```python
from build123d import *

# Parameters (mm, degrees)
SKETCH1_R           = 7.5
SKETCH1_R_2         = 3
BOSS_EXTRUDE1_DEPTH = 12.7


with BuildPart() as part:
    # Sketch1 → Boss-Extrude1 (new body)
    with BuildSketch(Plane(origin=(0, 0, 0), x_dir=(1, 0, 0), z_dir=(0, 1, 0))):
        with BuildLine():
            Line((4.628728323, 75), (-4.628728323, 75))
            ThreePointArc((-4.628728323, 75), (-8.298056729, 73.747212766), (-10.435089207, 70.512009682))
            add(Edge.make_bspline(
                [(-10.435089207, 70.512009682), (-11.436889623, 66.664934619), (-14.691827535, 59.170334198), (-20.319154818, 53.251718644), (-23.989109736, 50.544662785)],
                knots=[0.130554933, 0.130554933, 0.130554933, 0.130554933, 0.477565762, 0.872598063, 0.872598063, 0.872598063, 0.872598063], degree=3))
            ThreePointArc((-23.989109736, 50.544662785), (-26.161679176, 47.482134252), (-26.088483789, 43.727965713))
            add(Edge.make_bspline(
                [(-26.088483789, 43.727965713), (-23.983802584, 37.735198712), (-21.861167747, 26.954437426), (-23.911988058, 18.58322157), (-25.980762, 15)],
                knots=[0.052697527, 0.052697527, 0.052697527, 0.052697527, 0.276348764, 0.5, 0.5, 0.5, 0.5], degree=3))
            add(Edge.make_bspline(
                [(-50.913771074, 0.729306865), (-44.671541988, 1.902983), (-34.273811388, 5.455107991), (-28.049535938, 11.416778424), (-25.980762, 15)],
                knots=[0.052697527, 0.052697527, 0.052697527, 0.052697527, 0.276348763, 0.5, 0.5, 0.5, 0.5], degree=3))
            ThreePointArc((-50.913771074, 0.729306865), (-54.201574082, -1.084388344), (-55.767516863, -4.497152931))
            add(Edge.make_bspline(
                [(-66.282736261, -26.218952497), (-63.451971733, -23.427830356), (-58.58892633, -16.861671221), (-56.276918547, -9.028955057), (-55.767516863, -4.497152931)],
                knots=[0.130554933, 0.130554933, 0.130554933, 0.130554933, 0.477565762, 0.872598064, 0.872598064, 0.872598064, 0.872598064], degree=3))
            ThreePointArc((-66.282736261, -26.218952497), (-68.015988078, -29.687278454), (-67.266269445, -33.491403685))
            Line((-67.266269445, -33.491403685), (-62.637541122, -41.508596315))
            add(Edge.make_bspline(
                [(-62.637541122, -41.508596315), (-60.110445807, -44.518882553), (-55.847647053, -44.293057185)],
                knots=[0, 0, 0, 1, 1, 1], degree=2))
            Line((-55.847647053, -44.293057185), (55.847647053, -44.293057185))
            add(Edge.make_bspline(
                [(62.637541122, -41.508596315), (60.110445807, -44.518882553), (55.847647053, -44.293057185)],
                knots=[0, 0, 0, 1, 1, 1], degree=2))
            Line((62.637541122, -41.508596315), (67.266269445, -33.491403685))
            ThreePointArc((67.266269445, -33.491403685), (68.015988078, -29.687278454), (66.282736261, -26.218952497))
            add(Edge.make_bspline(
                [(66.282736261, -26.218952497), (63.451971733, -23.427830356), (58.58892633, -16.861671221), (56.276918547, -9.028955057), (55.767516863, -4.497152931)],
                knots=[0.130554933, 0.130554933, 0.130554933, 0.130554933, 0.477565762, 0.872598064, 0.872598064, 0.872598064, 0.872598064], degree=3))
            ThreePointArc((55.767516863, -4.497152931), (54.201574082, -1.084388344), (50.913771074, 0.729306865))
            add(Edge.make_bspline(
                [(50.913771074, 0.729306865), (44.671541988, 1.902983), (34.273811388, 5.455107991), (28.049535938, 11.416778424), (25.980762, 15)],
                knots=[0.052697527, 0.052697527, 0.052697527, 0.052697527, 0.276348763, 0.5, 0.5, 0.5, 0.5], degree=3))
            add(Edge.make_bspline(
                [(26.088483789, 43.727965713), (23.983802584, 37.735198712), (21.861167747, 26.954437426), (23.911988058, 18.58322157), (25.980762, 15)],
                knots=[0.052697527, 0.052697527, 0.052697527, 0.052697527, 0.276348764, 0.5, 0.5, 0.5, 0.5], degree=3))
            ThreePointArc((26.088483789, 43.727965713), (26.161679176, 47.482134252), (23.989109736, 50.544662785))
            add(Edge.make_bspline(
                [(10.435089207, 70.512009682), (11.436889623, 66.664934619), (14.691827535, 59.170334198), (20.319154818, 53.251718644), (23.989109736, 50.544662785)],
                knots=[0.130554933, 0.130554933, 0.130554933, 0.130554933, 0.477565762, 0.872598063, 0.872598063, 0.872598063, 0.872598063], degree=3))
            ThreePointArc((10.435089207, 70.512009682), (8.298056729, 73.747212766), (4.628728323, 75))
        make_face()
        with Locations(Location((0, 0, 0), (0, 0, 270))):
            Circle(SKETCH1_R, mode=Mode.SUBTRACT)
        with Locations(Location((0, 65, 0), (0, 0, 270))):
            Circle(SKETCH1_R_2, mode=Mode.SUBTRACT)
        with Locations(Location((0, 45, 0), (0, 0, 270))):
            Circle(SKETCH1_R_2, mode=Mode.SUBTRACT)
        with Locations(Location((56.291651246, -32.5, 0), (0, 0, 270))):
            Circle(SKETCH1_R_2, mode=Mode.SUBTRACT)
        with Locations(Location((38.97114317, -22.5, 0), (0, 0, 270))):
            Circle(SKETCH1_R_2, mode=Mode.SUBTRACT)
        with Locations(Location((-56.291651246, -32.5, 0), (0, 0, 270))):
            Circle(SKETCH1_R_2, mode=Mode.SUBTRACT)
        with Locations(Location((-38.97114317, -22.5, 0), (0, 0, 270))):
            Circle(SKETCH1_R_2, mode=Mode.SUBTRACT)
        with Locations(Location((-15.075454508, -18, 0), (0, 0, 270))):
            Circle(SKETCH1_R_2, mode=Mode.SUBTRACT)
        with Locations(Location((-15.075454508, -38, 0), (0, 0, 270))):
            Circle(SKETCH1_R_2, mode=Mode.SUBTRACT)
        with Locations(Location((14.924545492, -38, 0), (0, 0, 270))):
            Circle(SKETCH1_R_2, mode=Mode.SUBTRACT)
        with Locations(Location((14.924545492, -18, 0), (0, 0, 270))):
            Circle(SKETCH1_R_2, mode=Mode.SUBTRACT)
    extrude(amount=BOSS_EXTRUDE1_DEPTH)


solid = part.part
```
Verification items for the finished model (mm, model axes). Coordinates: 2 decimals unless noted, no trailing zeros. Order: outer loops, then holes, each group sorted by start corner. A loop starts at its lowest first (then second) coordinate and runs counter-clockwise, first axis right, second up. Notation, with made-up numbers: (65.25, 48) - (102.25, 48) arc R14 ccw to (102.25, 67) - close; hole circle Ø11 at (34.5, 7.5). An arc over 180 degrees is marked (long way). Return JSON: item names as keys, results as strings.
(1) Mould release check, pull along X, two halves, no side actions. Record for faces 1 (the cylindrical face through (-8.254, 6.261, -73.781)), 2 (the flat face through (0, 6, -75)), 3 (the cylindrical face through (-15, 6, 35)): pulls with the +X half, pulls with the -X half, needs draft (parallel to the pull), parting line crosses it, or undercut.
Filled sheet:
{"face 1": "pulls with the -X half", "face 2": "needs draft", "face 3": "undercut"}
(2) Thickness scan on line 1 along X through (y, z) = (8.5, 18); line 2 along X through (y, z) = (2.75, -65); line 3 along Z through (x, y) = (55, 4.75). Record the ranges inside material, lowest first.
Filled sheet:
{"line 1": "x = -59.99 to -18.08, -12.08 to 11.92, 17.92 to 59.99", "line 2": "x = -12.33 to -3, 3 to 12.33", "line 3": "z = 2.17 to 29.79, 35.21 to 44.29"}
(3) Section check C-C, the plane z = 1. Record the cut outline in (x, y).
Filled sheet:
{"outline": "(-54.12, 0) - (-7.43, 0) - (-7.43, 12.7) - (-54.12, 12.7) - close; (7.43, 0) - (54.12, 0) - (54.12, 12.7) - (7.43, 12.7) - close"}
(4) Section check B-B, the plane z = 38. Record the cut outline in (x, y), and give its area (3 significant figures).
Filled sheet:
{"outline": "(-64.66, 0) - (-18.08, 0) - (-18.08, 12.7) - (-64.66, 12.7) - close; (-12.08, 0) - (11.92, 0) - (11.92, 12.7) - (-12.08, 12.7) - close; (17.92, 0) - (64.66, 0) - (64.66, 12.7) - (17.92, 12.7) - close", "area": "1,490 mm^2"}
(5) Section check A-A, the plane x = 0. Record the cut outline in (y, z), and give its area (3 significant figures).
Filled sheet:
{"outline": "(0, -75) - (12.7, -75) - (12.7, -68) - (0, -68) - close; (0, -62) - (12.7, -62) - (12.7, -48) - (0, -48) - close; (0, -42) - (12.7, -42) - (12.7, -7.5) - (0, -7.5) - close; (0, 7.5) - (12.7, 7.5) - (12.7, 44.29) - (0, 44.29) - close", "area": "1,170 mm^2"}
(6) Section check D-D, the plane y = 5.75. Give the number of separate pieces and of enclosed holes in the cut face, and give its area (3 significant figures).
Filled sheet:
{"separate pieces": "1", "enclosed holes": "11", "area": "8,460 mm^2"}
(7) Go/stop test with flat-tipped pins: pin 1 (1 mm diameter, centred on x = 6, y = 3, fed in from -Z); pin 2 (3 mm diameter, centred on y = 2, z = -12, fed in from +X); pin 3 (4 mm diameter, centred on x = 10.5, y = 9, fed in from +Z); pin 4 (3.5 mm diameter, centred on x = 56.29, z = 32.5, fed in from -Y). Record where each tip stops, or that it passes through.
Filled sheet:
{"pin 1": "stops at z = -74.94", "pin 2": "stops at x = 29.44", "pin 3": "stops at z = 44.29", "pin 4": "passes through"}
